The drawing under review shows one solid part. Ordinate dimensions are in mm from its lowest x, y, z. Coordinates: 2 decimals unless noted, no trailing zeros. Write each loop counter-clockwise with the first axis right and the second up, starting at its lowest first coordinate (ties: lowest second). Pieces come first, ordered by that corner, then holes.
1) For line 1 (X direction, y = 1.35, z = 78.35); line 2 (X direction, y = 0.4, z = 125.5); line 3 (Z direction, x = 124, y = 1.3), list the stretches that pass through material, from the lowest coordinate up.
2) Add section C-C, the plane y = 1.05. State the section outline as (x, z) points.
3) Add section D-D, the plane x = 78.35. State the section outline as (y, z) points, then the cut area to 3 significant figures.
4) Add section A-A, the plane z = 78.35. State the section outline as (x, y) points, then the cut area to 3 significant figures.
5) Add section B-B, the plane x = 15.85. State the section outline as (y, z) points.
6) For P1, Ø6.5, axis at x = 78.35, z = 15.85, coming from the -Y side; P2, Ø1, axis at y = 0.5, z = 118.5, coming from the -X side; P3, Ø0.9, axis at y = 1, z = 91.5, coming from the -X side; P4, Ø0.9, axis at x = 86.5, y = 1, coming from the +Z side, all flat-tipped, find the tip position at first contact; note any pin that passes through.
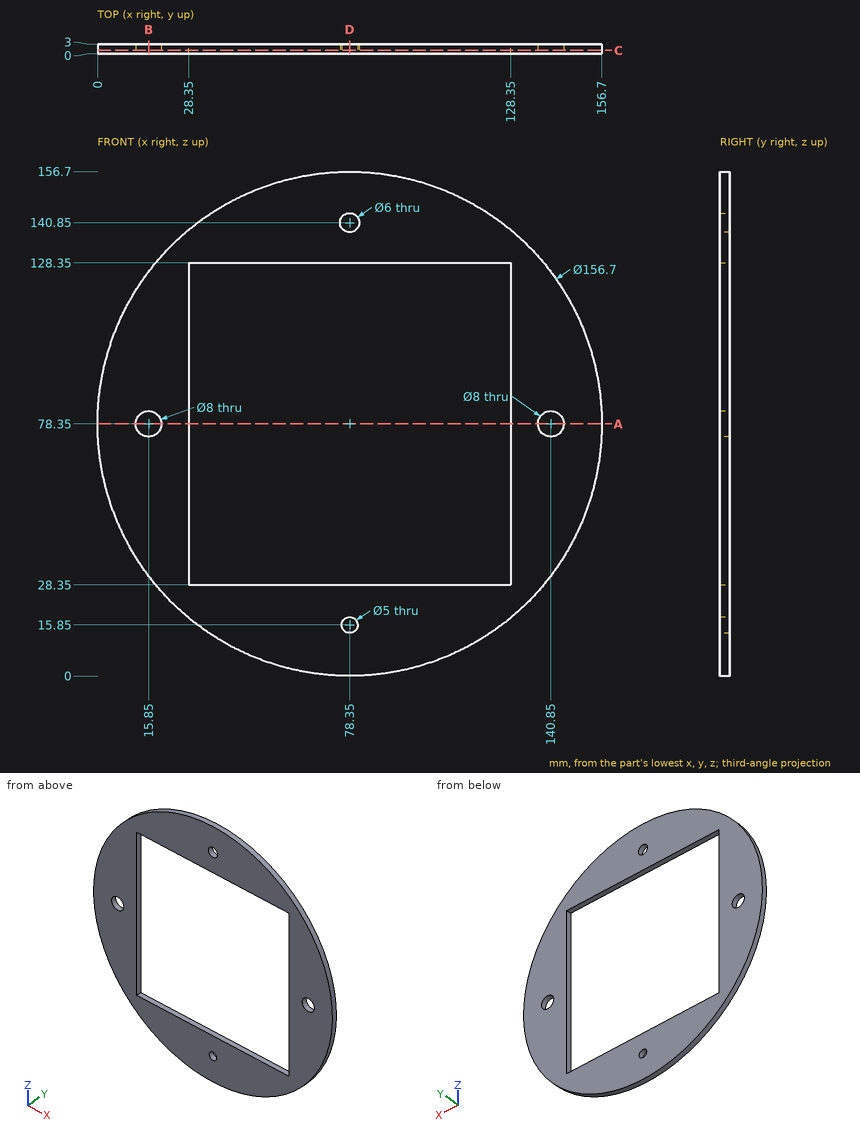
Geometry results:
1. line 1: x = 0 to 11.85, 19.85 to 28.35, 128.35 to 136.85, 144.85 to 156.7
1. line 2: x = 15.78 to 28.35, 128.35 to 140.92
1. line 3: z = 14.67 to 28.35, 128.35 to 142.03
2. outline: circle Ø156.7 at (78.35, 78.35); hole circle Ø8 at (15.85, 78.35); hole (28.35, 28.35) - (128.35, 28.35) - (128.35, 128.35) - (28.35, 128.35) - close; hole circle Ø6 at (78.35, 140.85); hole circle Ø5 at (78.35, 15.85); hole circle Ø8 at (140.85, 78.35)
3. outline: (0, 0) - (3, 0) - (3, 13.35) - (0, 13.35) - close; (0, 18.35) - (3, 18.35) - (3, 28.35) - (0, 28.35) - close; (0, 128.35) - (3, 128.35) - (3, 137.85) - (0, 137.85) - close; (0, 143.85) - (3, 143.85) - (3, 156.7) - (0, 156.7) - close
3. area: 137 mm2
4. outline: (0, 0) - (11.85, 0) - (11.85, 3) - (0, 3) - close; (19.85, 0) - (28.35, 0) - (28.35, 3) - (19.85, 3) - close; (128.35, 0) - (136.85, 0) - (136.85, 3) - (128.35, 3) - close; (144.85, 0) - (156.7, 0) - (156.7, 3) - (144.85, 3) - close
4. area: 122 mm2
5. outline: (0, 31.1) - (3, 31.1) - (3, 74.35) - (0, 74.35) - close; (0, 82.35) - (3, 82.35) - (3, 125.6) - (0, 125.6) - close
6. P1: stops at y = 0
6. P2: stops at x = 10.77
6. P3: stops at x = 1.04
6. P4: stops at z = 156.32
